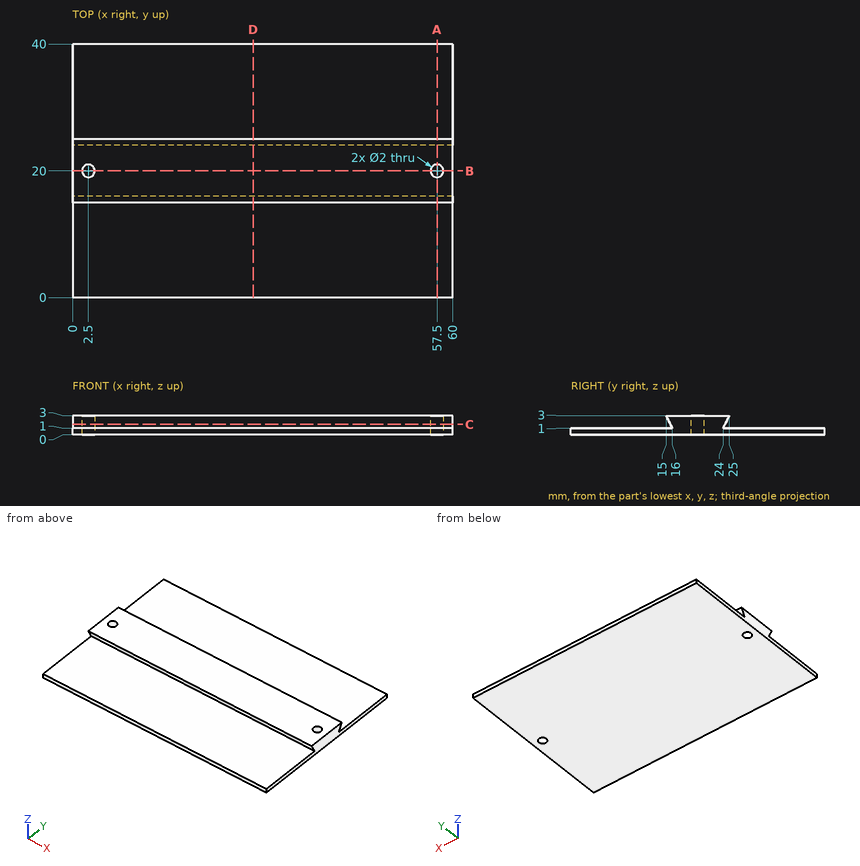
Geometry: see drawing. Coordinates: mm, zero at the bounding-box minimum. Round coordinates to 2 decimals unless told otherwise and drop trailing zeros. Order: outer loops, then holes, each group sorted by start corner. A loop starts at its lowest first (then second) coordinate and runs counter-clockwise, first axis right, second up. Notation, with made-up numbers: (7.5, 29.25) - (42.5, 29.25) arc R24 cw to (42.5, 55.25) - close; hole circle Ø2 at (38, -23.5). An arc over 180 degrees is marked (long way). Use a Markdown table: item, result. Add a question column.
1. Section query D-D (x = 28.5). Return the cut outline in (y, z), then the cut area to 3 significant figures.
2. Section query A-A (x = 57.5). Return the cut outline in (y, z), then the cut area to 3 significant figures.
3. Section query C-C (z = 1.6). Return the cut outline in (x, y).
4. Section query B-B (y = 20). Return the cut outline in (x, z).
5. Line query: probe 1 along Z at (x, y) = (22, 10.5); probe 2 along Z at (x, y) = (18.5, 15.5); probe 3 along Y at (x, z) = (57.5, 1.3). Output: solid intervals per line, ascending.
6. First-contact query: pin 1 (1.5 mm diameter, centred on x = 35.5, y = 33.5, fed in from +Z); pin 2 (2.5 mm diameter, centred on x = 57.5, y = 20, fed in from +Z). Flat tips, straight axial feed; report the tip coordinate or a pass-through.
Derived:
| question | item | result |
|---|---|---|
| 1 | outline | (0, 0) - (40, 0) - (40, 1) - (24, 1) - (25, 3) - (15, 3) - (16, 1) - (0, 1) - close |
| 1 | area | 58.0 mm2 |
| 2 | outline | (0, 0) - (19, 0) - (19, 3) - (15, 3) - (16, 1) - (0, 1) - close; (21, 0) - (40, 0) - (40, 1) - (24, 1) - (25, 3) - (21, 3) - close |
| 2 | area | 52.0 mm2 |
| 3 | outline | (0, 15.7) - (60, 15.7) - (60, 24.3) - (0, 24.3) - close; hole circle Ø2 at (2.5, 20); hole circle Ø2 at (57.5, 20) |
| 4 | outline | (0, 0) - (1.5, 0) - (1.5, 3) - (0, 3) - close; (3.5, 0) - (56.5, 0) - (56.5, 3) - (3.5, 3) - close; (58.5, 0) - (60, 0) - (60, 3) - (58.5, 3) - close |
| 5 | probe 1 | 0 to 1 |
| 5 | probe 2 | 0 to 1, 2 to 3 |
| 5 | probe 3 | 15.85 to 19, 21 to 24.15 |
| 6 | pin 1 | z = 1 |
| 6 | pin 2 | z = 3 |
